Design review of the part shown in the three views and the two pictorial views. Dimensions are in mm from the part's minimum x, y and z. A direction names the side the tool comes from. Coordinates: 2 decimals unless noted, no trailing zeros. Write each loop counter-clockwise with the first axis right and the second up, starting at its lowest first coordinate (ties: lowest second). Pieces come first, ordered by that corner, then holes. Notation, with made-up numbers: (-16, 65) -> (25, 65) arc R19 ccw to (25, 99) -> close; hole circle Ø2 at (-3, 59.25). An arc over 180 degrees is marked (long way). Write each question's results on one line, items separated by ' | '.
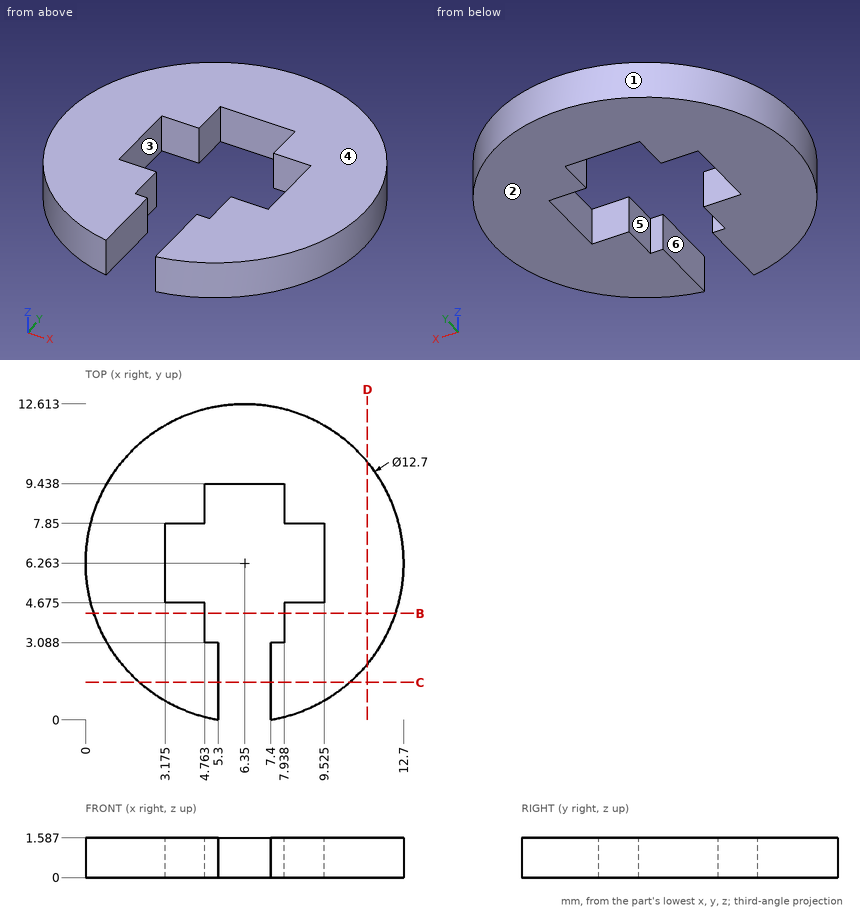
Q1. Draft analysis for pull direction Y (two halves, no side actions). For the marked faces 1, 2 and 3, state which applies: pulls with the +Y half, pulls with the -Y half, needs draft (parallel to the pull), parting line crosses it, or undercut.
Solution:
face 1: parting line crosses it | face 2: needs draft | face 3: undercut
Q2. Clearance check with flat-ended pins moving along their axes: P1, Ø0.8, axis at x = 9, z = 1, coming from the -Y side (1 decimal); P2, Ø0.8, axis at y = 9, z = 1, coming from the -X side (1 decimal); P3, Ø0.8, axis at y = 6, z = 1, coming from the -X side; P4, Ø0.8, axis at y = 1, z = 1, coming from the +X side (1 decimal). State where each tip first meets the part, or that it passes through.
Solution:
P1: y = 0.3 | P2: x = 0.4 | P3: x = 0 | P4: x = 10.4
Q3. For line 1 (X direction, y = 4.5, z = 0.95); line 2 (X direction, y = 7.75, z = 0.45) (1 decimal); line 3 (Y direction, x = 5.25, z = 1.2), list the stretches that pass through material, from the lowest coordinate up. Write a range as from..to.
Solution:
line 1: 0.25..4.76, 7.94..12.45 | line 2: 0.2..3.2, 9.5..12.5 | line 3: 0.01..3.09, 9.44..12.52
Q4. Add section B-B (y = 4.25). Write out the cut boundary in (x, z), plus the area to 3 significant figures.
Solution:
outline: (0.33, 0) -> (4.76, 0) -> (4.76, 1.59) -> (0.33, 1.59) -> close; (7.94, 0) -> (12.37, 0) -> (12.37, 1.59) -> (7.94, 1.59) -> close | area: 14.1 mm²
Q5. Add section C-C (y = 1.5). Write out the cut boundary in (x, z).
Solution:
outline: (2.15, 0) -> (5.3, 0) -> (5.3, 1.59) -> (2.15, 1.59) -> close; (7.4, 0) -> (10.55, 0) -> (10.55, 1.59) -> (7.4, 1.59) -> close
Q6. Add section D-D (x = 11.25). Write out the cut boundary in (y, z).
Solution:
outline: (2.22, 0) -> (10.3, 0) -> (10.3, 1.59) -> (2.22, 1.59) -> close
Q7. Machinability: for the marked faces 4, 5 and 6, which of the approach directions +Z, -Z, +X, -X, +Y, -Y give a long, thin tool a straight path to every point of the face, cutting with its end or side? Answer none if there is none.
Solution:
face 4: +Z, +X, -X, +Y, -Y | face 5: +Z, -Z | face 6: +Z, -Z, -Y
